Input: part model. Units: mm. Frame: model coordinates. Face numbers are marked on the shaded views. A direction names the side the tool comes from. Give positions to 0.01 mm unless a question says otherwise; leave off trailing zeros. Order: outer loops, then holes, each group sorted by start corner. A loop starts at its lowest first (then second) coordinate and runs counter-clockwise, first axis right, second up. Notation, with made-up numbers: (88.25, 69) - (144.25, 69) arc R12 ccw to (144.25, 73) - close; hole circle Ø1 at (-19, 56). An arc over 180 degrees is marked (long way). Use a Markdown table: item, result.
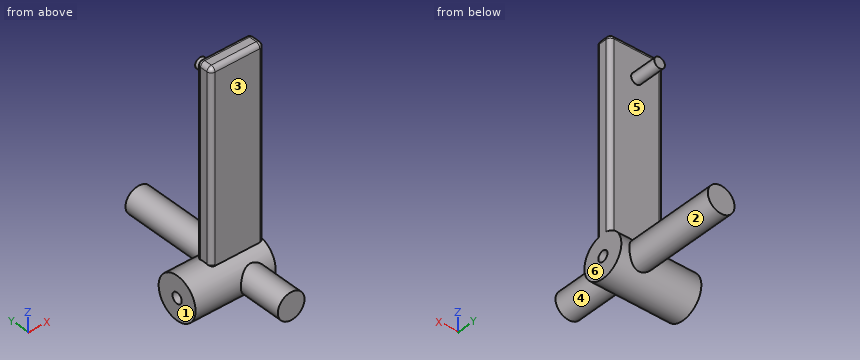
from build123d import *

# Parameters (mm, degrees)
SKETCH2_R                = 4
SKETCH2_R_2              = 1
BOSS_EXTRUDE1_DEPTH      = 15
SKETCH4_R                = 2.5
BOSS_EXTRUDE2_DEPTH      = 17
SKETCH6_R                = 2.5
BOSS_EXTRUDE3_DEPTH      = 16
SKETCH8_R                = 1
CUT_EXTRUDE1_DEPTH       = 27.115129868
SKETCH10_W               = 10
SKETCH10_H               = 3
BOSS_EXTRUDE4_DEPTH      = 35
FILLET1_R                = 0.8
BOSS_EXTRUDE5_REACH      = 45.486
BOSS_EXTRUDE5_END_RADIUS = 4
SKETCH12_R               = 1
BOSS_EXTRUDE6_DEPTH      = 5


with BuildPart() as part:
    # Sketch2 → Boss-Extrude1 (new body)
    with BuildSketch(Plane(origin=(0, 0, 0), x_dir=(0, 0, -1), z_dir=(1, 0, 0))):
        Circle(SKETCH2_R)
        Circle(SKETCH2_R_2, mode=Mode.SUBTRACT)
    extrude(amount=BOSS_EXTRUDE1_DEPTH)



with BuildPart() as body_2:
    # Sketch4 → Boss-Extrude2 (new body)
    with BuildSketch(Plane(origin=(15, 4, 0), x_dir=(1, 0, 0), z_dir=(0, 1, 0))):
        with Locations(Location((-4, 0, 0), (0, 0, 270))):
            Circle(SKETCH4_R)
    extrude(amount=BOSS_EXTRUDE2_DEPTH)


with BuildPart() as part_1:
    add(part.part)

    add(body_2.part)  # Boss-Extrude3 merges body 2
    # Sketch6 → Boss-Extrude3 (add)
    with BuildSketch(Plane.XZ.offset(-4)):
        with Locations(Location((11, 0, 0), (0, 0, 90))):
            Circle(SKETCH6_R)
    extrude(amount=BOSS_EXTRUDE3_DEPTH)

    # Sketch8 → Cut-Extrude1 (cut, through all)
    with BuildSketch(Plane(origin=(15, 0, 0), x_dir=(0, 0, -1), z_dir=(1, 0, 0))):
        Circle(SKETCH8_R)
    extrude(amount=-CUT_EXTRUDE1_DEPTH, mode=Mode.SUBTRACT)



with BuildPart() as body_2_2:
    # Sketch10 → Boss-Extrude4 (new body)
    with BuildSketch(Plane(origin=(15, 0, 4), x_dir=(1, 0, 0), z_dir=(0, 0, 1))):
        with Locations((-5, 0)):
            Rectangle(SKETCH10_W, SKETCH10_H)
    extrude(amount=BOSS_EXTRUDE4_DEPTH)

    # Fillet1
    fillet1_edges = [body_2_2.edges().sort_by_distance(p)[0] for p in [
        (10, -1.5, 39),
        (15, 0, 39),
        (10, 1.5, 39),
        (15, 1.5, 21.5),
        (15, -1.5, 21.5),
        (5, -1.5, 21.5),
        (5, 1.5, 21.5),
        (5, 0, 39),
    ]]
    fillet(fillet1_edges, radius=FILLET1_R)


with BuildPart() as part_2:
    add(part_1.part)

    add(body_2_2.part)  # Boss-Extrude5 merges body 2 2
    # Boss-Extrude5: up to this cylinder (the profile starts outside it)
    boss_extrude5_end = Plane(origin=(10, 0, 0), z_dir=(-1, 0, 0)) * Cylinder(BOSS_EXTRUDE5_END_RADIUS, 99.972, mode=Mode.PRIVATE)
    # Sketch11 → Boss-Extrude5 (add, up to the surface)
    with BuildSketch(Plane(origin=(15, 0, 4), x_dir=(1, 0, 0), z_dir=(0, 0, 1)), mode=Mode.PRIVATE) as boss_extrude5_sk1:
        with BuildLine():
            Line((-9.2, -1.5), (-0.8, -1.5))
            ThreePointArc((-0.8, -1.5), (-0.234314575, -1.265685425), (0, -0.7))
            Line((0, -0.7), (0, 0.7))
            ThreePointArc((0, 0.7), (-0.234314575, 1.265685425), (-0.8, 1.5))
            Line((-0.8, 1.5), (-9.2, 1.5))
            ThreePointArc((-9.2, 1.5), (-9.765685425, 1.265685425), (-10, 0.7))
            Line((-10, 0.7), (-10, -0.7))
            ThreePointArc((-10, -0.7), (-9.765685425, -1.265685425), (-9.2, -1.5))
        make_face()
    boss_extrude5_tool1 = extrude(boss_extrude5_sk1.sketch, amount=-BOSS_EXTRUDE5_REACH, mode=Mode.PRIVATE) - boss_extrude5_end
    add(boss_extrude5_tool1.solids().sort_by_distance((10, 0, 4))[0])
    add(boss_extrude5_tool1.solids().sort_by_distance((10, 0, 4))[1])

    # Sketch12 → Boss-Extrude6 (add)
    with BuildSketch(Plane(origin=(0, 1.5, 0), x_dir=(1, 0, 0), z_dir=(0, 1, 0))):
        with Locations((10, -33.2)):
            Circle(SKETCH12_R)
    extrude(amount=BOSS_EXTRUDE6_DEPTH)


solid = part_2.part
1. Set-up query: the marked faces 1, 2 and 3. Return all of +Z, -Z, +X, -X, +Y, -Y with unobstructed straight access to the full face (end or side cutting, diameter ignored); none if empty.
Response:
| item | result |
|---|---|
| face 1 | +Z, -Z, -X, +Y, -Y |
| face 2 | +Y |
| face 3 | +Z, +X, -X, -Y |
2. Section query B-B (y = 0). Return loops of the section in (x, z), then the cut area to 3 significant figures.
Response:
| item | result |
|---|---|
| outline | (0, -4) - (15, -4) - (15, -1) - (0, -1) - close; (0, 1) - (15, 1) - (15, 38.2) arc R0.8 ccw to (14.2, 39) - (5.8, 39) arc R0.8 ccw to (5, 38.2) - (5, 4) - (0, 4) - close |
| area | 440 mm^2 |
3. Material intervals for line 1 along Y through (x, z) = (9.85, 0); line 2 along Z through (x, y) = (13.7, 0); line 3 along Y through (x, z) = (3.75, 0), sorted ascending.
Response:
| item | result |
|---|---|
| line 1 | y = -12 to -1, 1 to 21 |
| line 2 | z = -4 to -1, 1 to 39 |
| line 3 | y = -4 to -1, 1 to 4 |
4. Section query C-C (z = 24.5). Return loops of the section in (x, y), then the cut area to 3 significant figures.
Response:
| item | result |
|---|---|
| outline | (5, -0.7) arc R0.8 ccw to (5.8, -1.5) - (14.2, -1.5) arc R0.8 ccw to (15, -0.7) - (15, 0.7) arc R0.8 ccw to (14.2, 1.5) - (5.8, 1.5) arc R0.8 ccw to (5, 0.7) - close |
| area | 29.5 mm^2 |
5. Section query D-D (x = 11.5). Return loops of the section in (y, z).
Response:
| item | result |
|---|---|
| outline | (-12, -2.45) - (-3.16, -2.45) arc R4 ccw to (3.16, -2.45) - (21, -2.45) - (21, 2.45) - (3.16, 2.45) arc R4 ccw to (1.5, 3.71) - (1.5, 38.2) arc R0.8 ccw to (0.7, 39) - (-0.7, 39) arc R0.8 ccw to (-1.5, 38.2) - (-1.5, 3.71) arc R4 ccw to (-3.16, 2.45) - (-12, 2.45) - close; hole circle Ø2 at (0, 0) |
6. Mould query, pull axis Z, two halves, no side actions, for the marked faces 4, 5 and 6. Classes: pulls with the +Z half, pulls with the -Z half, needs draft (parallel to the pull), parting line crosses it, or undercut.
Response:
| item | result |
|---|---|
| face 4 | parting line crosses it |
| face 5 | undercut |
| face 6 | needs draft |
7. Pin query (flat end, axial travel): pin 1 (8 mm diameter, centred on x = 6, y = 12.5, fed in from -Z); pin 2 (2.5 mm diameter, centred on x = 10, z = 21.5, fed in from -Y); pin 3 (2 mm diameter, centred on x = 2.5, y = -3.5, fed in from -Z). Return the tip coordinate at first contact, or that it passes through.
Response:
| item | result |
|---|---|
| pin 1 | stops at z = -2.29 |
| pin 2 | stops at y = -1.5 |
| pin 3 | stops at z = -3.12 |
8. Section query A-A (z = 0). Return loops of the section in (x, y), then the cut area to 3 significant figures.
Response:
| item | result |
|---|---|
| outline | (0, -4) - (8.5, -4) - (8.5, -12) - (13.5, -12) - (13.5, -4) - (15, -4) - (15, -1) - (0, -1) - close; (0, 1) - (15, 1) - (15, 4) - (13.5, 4) - (13.5, 21) - (8.5, 21) - (8.5, 4) - (0, 4) - close |
| area | 215 mm^2 |
